from build123d import *

# Parameters (mm, degrees)
SKETCH_1_R               = 2.05
EXTRUDE_1_DEPTH          = 2.5
PATTERN_CIRCULAR_1_COUNT = 12
CHAMFER_1_SIZE           = 0.5
CHAMFER_2_SIZE           = 0.5
CHAMFER_3_SIZE           = 0.3


with BuildPart() as part:
    # 스케치1 → 보스-돌출1 (new, symmetric)
    with BuildSketch(Plane.XY):
        with BuildLine():
            ThreePointArc((-0.75, 3.929058411), (0, -4), (0.75, 3.929058411))
            Line((0.75, 3.929058411), (0.659376088, 4.695031864))
            Line((0.659376088, 4.695031864), (0.5, 5.477225575))
            ThreePointArc((0.5, 5.477225575), (0, 5.5), (-0.5, 5.477225575))
            Line((-0.5, 5.477225575), (-0.659376088, 4.695031864))
            Line((-0.659376088, 4.695031864), (-0.75, 3.929058411))
        make_face()
        Circle(SKETCH_1_R, mode=Mode.SUBTRACT)
    extrude_1 = extrude(amount=EXTRUDE_1_DEPTH, both=True)

    # 원형 패턴1: 보스-돌출1 ×12 about axis
    pattern_circular_1_axis = Axis((0, 0, 0), (0, 0, 1))
    for i in range(1, PATTERN_CIRCULAR_1_COUNT):
        add(extrude_1.rotate(pattern_circular_1_axis, i * 360 / PATTERN_CIRCULAR_1_COUNT))

    # 모따기1
    chamfer_1_edges = [part.edges().sort_by_distance(p)[0] for p in [
        (0, 5.5, -2.5),
        (2.75, 4.763139721, -2.5),
        (5.5, 0, -2.5),
        (2.75, -4.763139721, -2.5),
        (-2.75, -4.763139721, -2.5),
        (-5.5, 0, -2.5),
        (-2.75, 4.763139721, -2.5),
        (-4.763139721, 2.75, -2.5),
        (-4.763139721, -2.75, -2.5),
        (0, -5.5, -2.5),
        (4.763139721, -2.75, -2.5),
        (4.763139721, 2.75, -2.5),
    ]]
    chamfer(chamfer_1_edges, length=CHAMFER_1_SIZE)

    # 모따기2
    chamfer_2_edges = [part.edges().sort_by_distance(p)[0] for p in [
        (4.763139721, 2.75, 2.5),
        (2.75, 4.763139721, 2.5),
        (0, 5.5, 2.5),
        (-2.75, 4.763139721, 2.5),
        (-4.763139721, 2.75, 2.5),
        (-5.5, 0, 2.5),
        (-4.763139721, -2.75, 2.5),
        (-2.75, -4.763139721, 2.5),
        (0, -5.5, 2.5),
        (2.75, -4.763139721, 2.5),
        (4.763139721, -2.75, 2.5),
        (5.5, 0, 2.5),
    ]]
    chamfer(chamfer_2_edges, length=CHAMFER_2_SIZE)

    # 모따기3
    chamfer_3_edges = [part.edges().sort_by_distance(p)[0] for p in [
        (-2.05, 0, 2.5),
        (-2.05, 0, -2.5),
    ]]
    chamfer(chamfer_3_edges, length=CHAMFER_3_SIZE)


solid = part.part
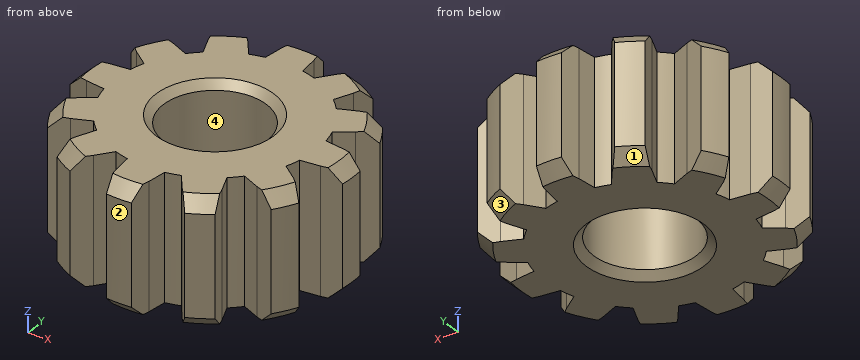
Part model, mm, in its own coordinate system. Face numbers are marked on the shaded views. Round coordinates to 2 decimals unless told otherwise and drop trailing zeros. Order: outer loops, then holes, each group sorted by start corner. A loop starts at its lowest first (then second) coordinate and runs counter-clockwise, first axis right, second up. Notation, with made-up numbers: (8.25, 35.25) -> (47.25, 35.25) arc R16 ccw to (47.25, 52.25) -> close; hole circle Ø11 at (-11, -27.75). An arc over 180 degrees is marked (long way). Put each result on its own line as item: value.
Q1. Band-saw the part on A-A (x = 0). Give the cut face in (y, z).
From the geometry:
outline: (-5.5, -2) -> (-5, -2.5) -> (-2.35, -2.5) -> (-2.05, -2.2) -> (-2.05, 2.2) -> (-2.35, 2.5) -> (-5, 2.5) -> (-5.5, 2) -> close; (2.05, -2.2) -> (2.35, -2.5) -> (5, -2.5) -> (5.5, -2) -> (5.5, 2) -> (5, 2.5) -> (2.35, 2.5) -> (2.05, 2.2) -> close
Q2. Wall check: line 1 (Y direction, x = 0, z = 1); line 2 (Y direction, x = -2.75, z = -2.1); line 3 (X direction, y = 4.25, z = -0.8). Give the ranges that are in metal, low to high. Write a range as [from, to].
From the geometry:
line 1: y = [-5.5, -2.05], [2.05, 5.5]
line 2: y = [-4.65, -3.34], [-2.9, 2.9], [3.34, 4.65]
line 3: x = [-3.09, -1.67], [-0.71, 0.71], [1.67, 3.09]
Q3. Pull direction X, two halves, no side cores. Call the marked faces 1, 2, 3 and 4: pulls with the +X half, pulls with the -X half, needs draft (parallel to the pull), parting line crosses it, or undercut.
From the geometry:
face 1: pulls with the -X half
face 2: parting line crosses it
face 3: pulls with the +X half
face 4: undercut
Q4. Pin check, flat tips, straight feed: pin 1 Ø2 at (x, z) = (-4, 0.5) entering from -Y; pin 2 Ø5.5 at (x, y) = (0, 0) entering from -Z; pin 3 Ø1.5 at (x, z) = (4, 0) entering from -Y. Stop position of each tip, or through.
From the geometry:
pin 1: stops at y = -4.61
pin 2: stops at z = -2.5
pin 3: stops at y = -3.17
Q5. Band-saw the part on C-C (y = -4.25). State how many separate pieces and enclosed holes the cut face has, and give its area (3 significant figures).
From the geometry:
separate pieces: 3
enclosed holes: 0
area: 21.1 mm2
